Source: three-view drawing plus pictorial views. Frame: mm from the lowest corner of the part. A direction names the side the tool comes from. Give positions to 0.01 mm unless a question says otherwise; leave off trailing zeros. Order: outer loops, then holes, each group sorted by start corner. A loop starts at its lowest first (then second) coordinate and runs counter-clockwise, first axis right, second up. Notation, with made-up numbers: (26, -30.75) - (55, -30.75) arc R24 ccw to (55, -5.75) - close; hole circle Ø2 at (-31, 36.25). An arc over 180 degrees is marked (long way). Answer in a Markdown table with one row per item. Add a question column.
1. Ray query, line 1 (Z direction, x = 2.75, y = 18.75); line 2 (Z direction, x = 12.5, y = 27.8); line 3 (Z direction, x = 12.5, y = 27.2). Return the intervals inside material, ascending. Write a range as [from, to].
2. Access query for the marked faces 5 and 6. Directions: +Z, -Z, +X, -X, +Y, -Y. A direction counts if a zero-diameter tool reaches every point of the face in a straight line with its end or side. Return the directions, or none.
3. Section query A-A on x = 12.5. Count the separate pieces of the cut face and the enclosed holes in it, and give its area (3 significant figures).
4. Mould query, pull axis X, two halves, no side actions, for the marked faces 1, 2, 3 and 4. Classes: released by +X, released by -X, zero draft, split by the parting line, or undercut.
5. Contact query for flat-ended pins moving along their axis: pin 1 (5 mm diameter, centred on x = 7, y = 17.5, fed in from -Z); pin 2 (6 mm diameter, centred on x = 4, y = 22.5, fed in from +Z); pin 3 (2 mm diameter, centred on x = 10, y = 4.5, fed in from +Z). Output: stop coordinate, or through.
6. Section query B-B on z = 20. Return loops of the section in (x, y).
7. Section query C-C on y = 10. Return loops of the section in (x, z).
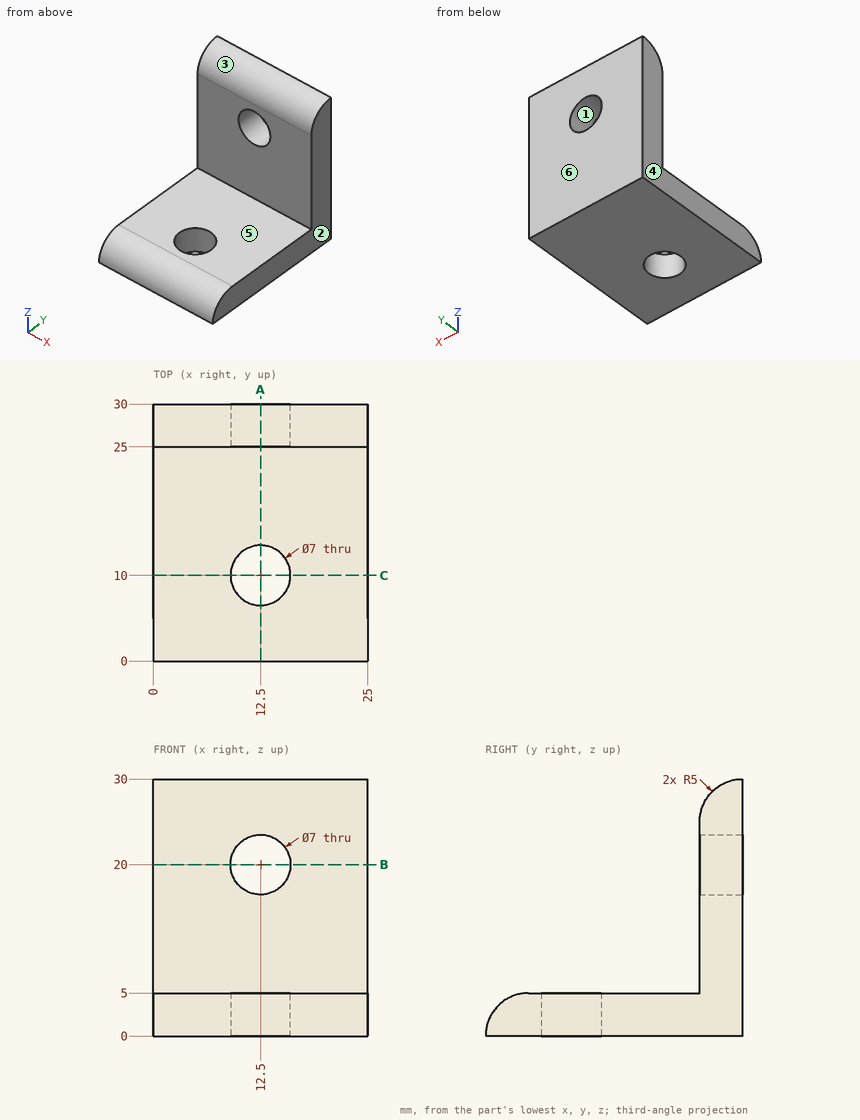
Answer:
| question | item | result |
|---|---|---|
| 1 | line 1 | z = [0, 5] |
| 1 | line 2 | z = [0, 16.5], [23.5, 29.49] |
| 1 | line 3 | z = [0, 16.5], [23.5, 29.14] |
| 2 | face 5 | +Z, +X, -X, -Y |
| 2 | face 6 | +Z, -Z, +X, -X, +Y |
| 3 | separate pieces | 3 |
| 3 | enclosed holes | 0 |
| 3 | area | 194 mm² |
| 4 | face 1 | undercut |
| 4 | face 2 | released by +X |
| 4 | face 3 | zero draft |
| 4 | face 4 | released by -X |
| 5 | pin 1 | stops at z = 0 |
| 5 | pin 2 | stops at z = 27.18 |
| 5 | pin 3 | stops at z = 5 |
| 6 | outline | (0, 25) - (9, 25) - (9, 30) - (0, 30) - close; (16, 25) - (25, 25) - (25, 30) - (16, 30) - close |
| 7 | outline | (0, 0) - (9, 0) - (9, 5) - (0, 5) - close; (16, 0) - (25, 0) - (25, 5) - (16, 5) - close |
